Could you check a few things on this drawing? It's one solid part, dimensions in mm from its lowest x, y, z. Give positions to 0.01 mm unless a question says otherwise; leave off trailing zeros. Write each loop counter-clockwise with the first axis right and the second up, starting at its lowest first coordinate (ties: lowest second). Pieces come first, ordered by that corner, then holes. Notation, with made-up numbers: (-22.5, 11) - (-7.5, 11) arc R3 cw to (-7.5, 16) - close; hole circle Ø6 at (62.25, -23.75). An arc over 180 degrees is marked (long way). One line per item, written item: value. Start each with the question number.
1) Please list where these lines run through material, in increasing order: L1, parallel to Y at x = 121, z = 0.65; L2, parallel to Y at x = 77, z = 0.9; L3, parallel to Y at x = 82.5, z = 0.4. Write a range as [from, to].
2) Imagine slicing it at C-C on z = 0.45. Write out the boundary of the cut face in (x, y), plus the area to 3 significant figures.
3) I'm going to push flat-ended pins straight in: P1, Ø3, axis at x = 121, y = 36.5, coming from the +Z side (3 decimals); P2, Ø3.5, axis at x = 5, y = 5, coming from the +Z side. Where does each tip first touch, or does it pass through?
4) Imagine slicing it at A-A on y = 36.5. Write out the boundary of the cut face in (x, z).
5) Imagine slicing it at B-B on x = 121. Write out the boundary of the cut face in (y, z), plus the area to 3 significant figures.
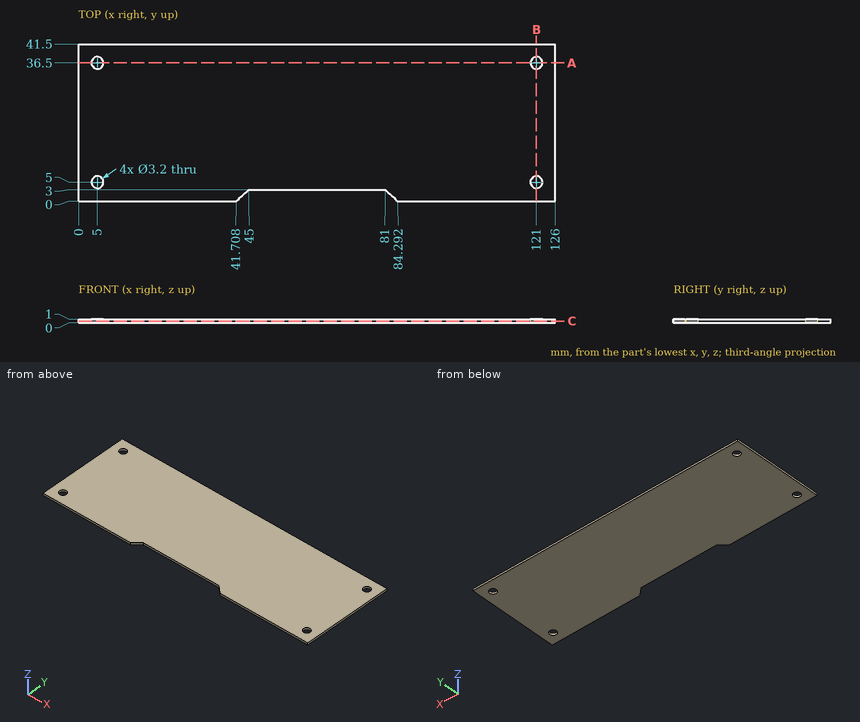
Numbers:
1. L1: [0, 3.4], [6.6, 34.9], [38.1, 41.5]
1. L2: [3, 41.5]
1. L3: [1.63, 41.5]
2. outline: (0, 0) - (41.71, 0) - (45, 3) - (81, 3) - (84.29, 0) - (126, 0) - (126, 41.5) - (0, 41.5) - close; hole circle Ø3.2 at (5, 5); hole circle Ø3.2 at (5, 36.5); hole circle Ø3.2 at (121, 5); hole circle Ø3.2 at (121, 36.5)
2. area: 5,080 mm^2
3. P1: through
3. P2: z = 1
4. outline: (0, 0) - (3.4, 0) - (3.4, 1) - (0, 1) - close; (6.6, 0) - (119.4, 0) - (119.4, 1) - (6.6, 1) - close; (122.6, 0) - (126, 0) - (126, 1) - (122.6, 1) - close
5. outline: (0, 0) - (3.4, 0) - (3.4, 1) - (0, 1) - close; (6.6, 0) - (34.9, 0) - (34.9, 1) - (6.6, 1) - close; (38.1, 0) - (41.5, 0) - (41.5, 1) - (38.1, 1) - close
5. area: 35.1 mm^2
